Verification items for the finished model (mm, model axes). Face numbers are marked on the shaded views. Round coordinates to 2 decimals unless told otherwise and drop trailing zeros. Loops run counter-clockwise (first coordinate to the right, second up) from the corner with the lowest first, then second, coordinate; pieces in that order, holes last. Notation, with made-up numbers: M 78.5,46.5 L 128.5,46.5 A17 ccw 128.5,51.5 Z; hole C 41.5,34.5 d8. An arc over 180 degrees is marked long. Answer as CSV lines item,"result".
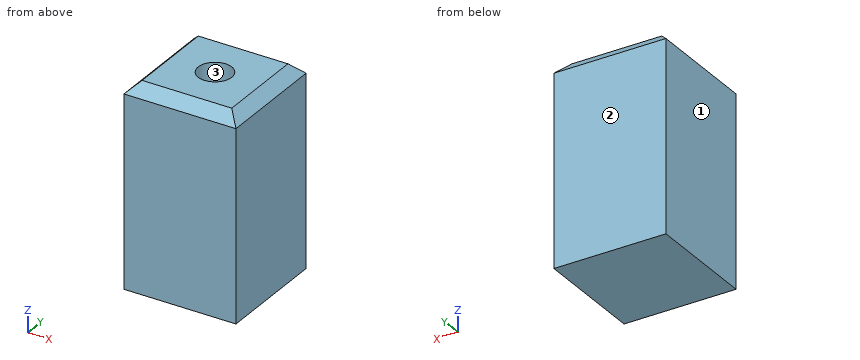
```python
from build123d import *

# Parameters (mm, degrees)
F0_W     = 50
F0_H     = 50
F1_DEPTH = 90
F2_SIZE  = 5
F4_R     = 7.5
F5_DEPTH = 20


with BuildPart() as f1:
    # F0 (on Top) → F1 (new body)
    with BuildSketch(Plane.XY):
        with Locations((-8.762377, -2.680112)):
            Rectangle(F0_W, F0_H)
    extrude(amount=F1_DEPTH)

    # F2
    f2_edges = [f1.edges().sort_by_distance(p)[0] for p in [
        (-8.762377, 22.319888, 90),
        (-33.762377, -2.680112, 90),
        (-8.762377, -27.680112, 90),
        (16.237623, -2.680112, 90),
    ]]
    chamfer(f2_edges, length=F2_SIZE)

    # F4 (on face) → F5 (cut)
    with BuildSketch(Plane.XY.offset(90)):
        with Locations((-8.762377, -2.680112)):
            Circle(F4_R)
    extrude(amount=-F5_DEPTH, mode=Mode.SUBTRACT)


solid = f1.part
```
1) Draft check along X on the marked faces 1, 2 and 3. Enter one of: +X half, -X half, draft (parallel to the pull), parting line (faces both ways), or undercut.
Here are the results:
face 1,"-X half"
face 2,"draft"
face 3,"undercut"
2) Material ranges on probe 1 along X at (y, z) = (2, 79); probe 2 along Z at (x, y) = (-9, -0.5); probe 3 along Y at (x, z) = (-10, 86.5), recorded low to high.
Here are the results:
probe 1,"x = -33.76 to -14.62, -2.9 to 16.24"
probe 2,"z = 0 to 70"
probe 3,"y = -26.18 to -10.08, 4.72 to 20.82"
3) Section check B-B (y = 3). Record the cut outline in (x, z).
Here are the results:
outline,"M -33.76,0 L 16.24,0 L 16.24,85 L 11.24,90 L -3.86,90 L -3.86,70 L -13.66,70 L -13.66,90 L -28.76,90 L -33.76,85 Z"
4) Section check C-C (z = 81). Record the cut outline in (x, y).
Here are the results:
outline,"M -33.76,-27.68 L 16.24,-27.68 L 16.24,22.32 L -33.76,22.32 Z; hole C -8.76,-2.68 d15"
5) Section check A-A (x = -12). Record the cut outline in (y, z), plus the area to 3 significant figures.
Here are the results:
outline,"M -27.68,0 L 22.32,0 L 22.32,85 L 17.32,90 L 4.09,90 L 4.09,70 L -9.45,70 L -9.45,90 L -22.68,90 L -27.68,85 Z"
area,"4,200 mm^2"
